```python
from build123d import *

# Parameters (mm, degrees)
EXTRU_MINCE1_DEPTH             = 32
EXTRU_MINCE1_DEPTH_BACK        = 32
BOSS_EXTRU_1_DEPTH             = 2
BOSS_EXTRU_1_DEPTH_BACK        = 0.1
ESQUISSE2_W                    = 4
ESQUISSE2_H                    = 2.5
ESQUISSE3_W                    = 31.28
ESQUISSE3_H                    = 65.9
ENL_V_MAT_EXTRU_4_DEPTH        = 1.75
ESQUISSE4_W                    = 4.5
ESQUISSE4_H                    = 6
BOSS_EXTRU_2_DEPTH             = 1
BOSS_EXTRU_3_REACH             = 40.572
BOSS_EXTRU_3_DIRECTION_2_REACH = 40.572
ENL_V_MAT_EXTRU_5_REACH        = 41.593
ESQUISSE7_W                    = 6.5
ESQUISSE7_H                    = 0.2
ESQUISSE7_W_2                  = 5.666666666
ESQUISSE7_W_3                  = 4.833333334
ESQUISSE7_W_4                  = 4
EXTRU_MINCE2_DEPTH             = 0.2
ESQUISSE8_R                    = 2.5
ENL_V_MAT_EXTRU_6_DEPTH        = 40.545037615
ESQUISSE9_R                    = 3.2
ESQUISSE9_R_2                  = 1.25
BOSS_EXTRU_4_DEPTH             = 1
CONG_1_R                       = 1


with BuildPart() as part:
    # Esquisse1 → Extru.-Mince1 (new, two sides: drawn at the far end of the back side and taken through both)
    with BuildSketch(Plane.XY.offset(-EXTRU_MINCE1_DEPTH_BACK)):
        with BuildLine():
            Line((-16.6, 0), (-16.6, -4.5))
            ThreePointArc((-16.6, -4.5), (-15.721320344, -6.621320344), (-13.6, -7.5))
            Line((-13.6, -7.5), (13.6, -7.5))
            ThreePointArc((13.6, -7.5), (15.721320344, -6.621320344), (16.6, -4.5))
            Line((16.6, -4.5), (16.6, 0))
            Line((16.6, 0), (14.89, 0))
            Line((14.89, 0), (14.89, -4.5))
            ThreePointArc((14.89, -4.5), (14.512167748, -5.412167748), (13.6, -5.79))
            Line((13.6, -5.79), (-13.6, -5.79))
            ThreePointArc((-13.6, -5.79), (-14.512167748, -5.412167748), (-14.89, -4.5))
            Line((-14.89, -4.5), (-14.89, 0))
            Line((-14.89, 0), (-16.6, 0))
        make_face()
    extrude(amount=EXTRU_MINCE1_DEPTH + EXTRU_MINCE1_DEPTH_BACK)

    # Esquisse2 → Boss.-Extru.1 (add, two sides: drawn at the far end of the back side and taken through both)
    with BuildSketch(Plane.XY.offset(32).offset(-BOSS_EXTRU_1_DEPTH_BACK)):
        with BuildLine():
            Line((16.6, -4.5), (16.6, 0))
            Line((16.6, 0), (3.5, 0))
            Line((3.5, 0), (3.5, 4))
            Line((3.5, 4), (-3.5, 4))
            Line((-3.5, 4), (-3.5, 0))
            Line((-3.5, 0), (-16.6, 0))
            Line((-16.6, 0), (-16.6, -4.5))
            ThreePointArc((-16.6, -4.5), (-15.721320344, -6.621320344), (-13.6, -7.5))
            Line((-13.6, -7.5), (13.6, -7.5))
            ThreePointArc((13.6, -7.5), (15.721320344, -6.621320344), (16.6, -4.5))
        make_face()
        with Locations((0, 1.25)):
            Rectangle(ESQUISSE2_W, ESQUISSE2_H, mode=Mode.SUBTRACT)
    extrude(amount=BOSS_EXTRU_1_DEPTH + BOSS_EXTRU_1_DEPTH_BACK)

    # Esquisse3 → Enlèv. mat.-Extru.4 (cut)
    with BuildSketch(Plane(origin=(0, 0, 0), x_dir=(1, 0, 0), z_dir=(0, 1, 0))):
        with Locations((0, 1.05)):
            Rectangle(ESQUISSE3_W, ESQUISSE3_H)
    extrude(amount=-ENL_V_MAT_EXTRU_4_DEPTH, mode=Mode.SUBTRACT)

    # Esquisse4 → Boss.-Extru.2 (add)
    with BuildSketch(Plane(origin=(0, -5.79, 0), x_dir=(1, 0, 0), z_dir=(0, 1, 0))):
        with Locations((0, 31)):
            Rectangle(ESQUISSE4_W, ESQUISSE4_H)
    extrude(amount=BOSS_EXTRU_2_DEPTH)

    # Boss.-Extru.3: up to this face of the body (flat: up to its plane)
    boss_extru_3_end = Plane(part.part.faces().sort_by_distance((2.25, -5.29, -31))[0])
    # Esquisse5 → Boss.-Extru.3 (add, up to the picked face)
    with BuildSketch(Plane(origin=(0, 0, 0), x_dir=(0, 0, -1), z_dir=(1, 0, 0)), mode=Mode.PRIVATE) as boss_extru_3_sk1:
        Polygon((34, -5.79), (34, -5.99), (33.8, -5.79), align=None)
    boss_extru_3_tool1 = split(extrude(boss_extru_3_sk1.sketch, amount=BOSS_EXTRU_3_REACH, mode=Mode.PRIVATE), bisect_by=boss_extru_3_end, keep=Keep.BOTH, mode=Mode.PRIVATE)
    add(boss_extru_3_tool1.solids().sort_by(Axis((0, -5.856667, -33.933333), (1, 0, 0)))[0])

    # Boss.-Extru.3 direction 2: up to this face of the body (flat: up to its plane)
    boss_extru_3_direction_2_end = Plane(part.part.faces().sort_by_distance((-2.25, -5.29, -31))[0])
    # Esquisse5 → Boss.-Extru.3 direction 2 (add, up to the picked face)
    with BuildSketch(Plane(origin=(0, 0, 0), x_dir=(0, 0, -1), z_dir=(1, 0, 0)), mode=Mode.PRIVATE) as boss_extru_3_direction_2_sk1:
        Polygon((34, -5.79), (34, -5.99), (33.8, -5.79), align=None)
    boss_extru_3_direction_2_tool1 = split(extrude(boss_extru_3_direction_2_sk1.sketch, amount=-BOSS_EXTRU_3_DIRECTION_2_REACH, mode=Mode.PRIVATE), bisect_by=boss_extru_3_direction_2_end, keep=Keep.BOTH, mode=Mode.PRIVATE)
    add(boss_extru_3_direction_2_tool1.solids().sort_by(Axis((0, -5.856667, -33.933333), (-1, 0, 0)))[0])

    # Esquisse6 → Enlèv. mat.-Extru.5 (cut, up to next)
    with BuildSketch(Plane(origin=(2.25, 0, 0), x_dir=(0, 0, -1), z_dir=(1, 0, 0)), mode=Mode.PRIVATE) as enl_v_mat_extru_5_sk1:
        Polygon((28, -5.79), (30, -4.79), (28, -4.79), align=None)
    enl_v_mat_extru_5_tool1 = extrude(enl_v_mat_extru_5_sk1.sketch, amount=-ENL_V_MAT_EXTRU_5_REACH, mode=Mode.PRIVATE) & part.part
    add(enl_v_mat_extru_5_tool1.solids().sort_by_distance((2.25, -5.123333, -28.666667))[0], mode=Mode.SUBTRACT)

    # Esquisse7 → Extru.-Mince2 (add)
    with BuildSketch(Plane.XZ.offset(7.5)):
        with Locations((0, -24.1)):
            Rectangle(ESQUISSE7_W, ESQUISSE7_H)
        with Locations((0, -22.6)):
            Rectangle(ESQUISSE7_W_2, ESQUISSE7_H)
        with Locations((0, -21.1)):
            Rectangle(ESQUISSE7_W_3, ESQUISSE7_H)
        with Locations((0, -19.6)):
            Rectangle(ESQUISSE7_W_4, ESQUISSE7_H)
    extrude(amount=EXTRU_MINCE2_DEPTH)

    # Esquisse8 → Enlèv. mat.-Extru.6 (cut, through all)
    with BuildSketch(Plane.XZ.offset(7.5)):
        with Locations((9.6, 27.5)):
            Circle(ESQUISSE8_R)
    extrude(amount=-ENL_V_MAT_EXTRU_6_DEPTH, mode=Mode.SUBTRACT)

    # Esquisse9 → Boss.-Extru.4 (add)
    with BuildSketch(Plane(origin=(0, -5.79, 0), x_dir=(1, 0, 0), z_dir=(0, 1, 0))):
        with Locations((9.6, -27.5)):
            Circle(ESQUISSE9_R)
        with Locations(Location((9.6, -27.5, 0), (0, 0, 180))):
            Circle(ESQUISSE9_R_2, mode=Mode.SUBTRACT)
    extrude(amount=BOSS_EXTRU_4_DEPTH)

    # Congé1
    cong_1_edges = [part.edges().sort_by_distance(p)[0] for p in [
        (15.721320344, -6.621320344, 34),
        (16.6, -2.25, 34),
        (-16.6, -2.25, 34),
        (-15.721320344, -6.621320344, 34),
        (0, -7.5, 34),
    ]]
    fillet(cong_1_edges, radius=CONG_1_R)


solid = part.part
```
Build history of the part. All positions in model axes, mm. A direction names the side the tool comes from. Coordinates: 2 decimals unless noted, no trailing zeros. Write each loop counter-clockwise with the first axis right and the second up, starting at its lowest first coordinate (ties: lowest second). Pieces come first, ordered by that corner, then holes.
1. Band-saw the part on B-B, the plane z = 27.5. Give the cut face in (x, y).
Answer block:
outline: (-16.6, -4.5) arc R3 ccw to (-13.6, -7.5) - (7.1, -7.5) - (7.1, -5.79) - (8.35, -5.79) - (8.35, -4.79) - (6.4, -4.79) - (6.4, -5.79) - (-13.6, -5.79) arc R1.29 cw to (-14.89, -4.5) - (-14.89, -1.75) - (-15.64, -1.75) - (-15.64, 0) - (-16.6, 0) - close; (10.85, -5.79) - (12.1, -5.79) - (12.1, -7.5) - (13.6, -7.5) arc R3 ccw to (16.6, -4.5) - (16.6, 0) - (15.64, 0) - (15.64, -1.75) - (14.89, -1.75) - (14.89, -4.5) arc R1.29 cw to (13.6, -5.79) - (12.8, -5.79) - (12.8, -4.79) - (10.85, -4.79) - close
2. Drop flat-ended pins along their axis: pin 1 (0.6 mm diameter, centred on x = 1, z = 33, fed in from -Y); pin 2 (1.3 mm diameter, centred on y = -5.5, z = -30, fed in from +X); pin 3 (1.1 mm diameter, centred on y = 1.5, z = 33, fed in from -X); pin 4 (1 mm diameter, centred on y = 2, z = -4, fed in from -X). Give the stop position or say it passes through.
Answer block:
pin 1: stops at y = -7.5
pin 2: stops at x = 16.58
pin 3: stops at x = -3.5
pin 4: passes through
3. Band-saw the part on A-A, the plane y = 1.5. Give the cut face in (x, z), and give its area (3 significant figures).
Answer block:
outline: (-3.5, 31.9) - (-2, 31.9) - (-2, 34) - (-3.5, 34) - close; (2, 31.9) - (3.5, 31.9) - (3.5, 34) - (2, 34) - close
area: 6.30 mm2
4. 3-axis set-ups, long thin cutter, end or side, ignore diameter. For faces 1 (the flat face through (16, 0, 11)), 2 (the flat face through (14.89, -3, 0)), 3 (the flat face through (-16, 0, 11)), 4 (the flat face through (-2, 1, 33)): which of +Z, -Z, +X, -X, +Y, -Y reach the whole face in a straight line?
Answer block:
face 1: +Z, -Z, +X, +Y
face 2: -Z, +Y
face 3: +Z, -Z, -X, +Y
face 4: +Z, -Z
5. Pull direction Z, two halves, no side cores. Call faces 5 (the cylindrical face through (9.27, -6.66, 29.98)), 6 (the cylindrical face through (9.87, -5.3, 26.28)), 7 (the cylindrical face through (-14.502, -5.422, -0.497)): released by +Z, released by -Z, zero draft, split by the parting line, or undercut.
Answer block:
face 5: undercut
face 6: undercut
face 7: zero draft
6. Band-saw the part on D-D, the plane x = -9. Give the cut face in (y, z), and give its area (3 significant figures).
Answer block:
outline: (-7.5, -32) - (-5.79, -32) - (-5.79, 31.9) - (0, 31.9) - (0, 34) - (-6.5, 34) arc R1 ccw to (-7.5, 33) - close
area: 125 mm2
7. Drill centre lines: probe 1 along Z at (x, y) = (9.6, -5.45); probe 2 along X at (y, z) = (-4.5, 17.5); probe 3 along X at (y, z) = (-1, -18.5). Where is each one in solid material? Low to high.
Answer block:
probe 1: z = 24.3 to 26.25, 28.75 to 30.7, 31.9 to 34
probe 2: x = -16.6 to -14.89, 14.89 to 16.6
probe 3: x = -16.6 to -15.64, 15.64 to 16.6
